For this review, take the finished solid that the model builds, in its own axes (mm). Face numbers are marked on the shaded views. A direction names the side the tool comes from. Coordinates: 2 decimals unless noted, no trailing zeros. Loops run counter-clockwise (first coordinate to the right, second up) from the corner with the lowest first, then second, coordinate; pieces in that order, holes last. Notation, with made-up numbers: (4, 47) -> (50, 47) arc R18 ccw to (50, 56) -> close; hole circle Ø4 at (9.5, -18.5). An arc over 180 degrees is marked (long way). Answer in a Markdown table with one row per item.
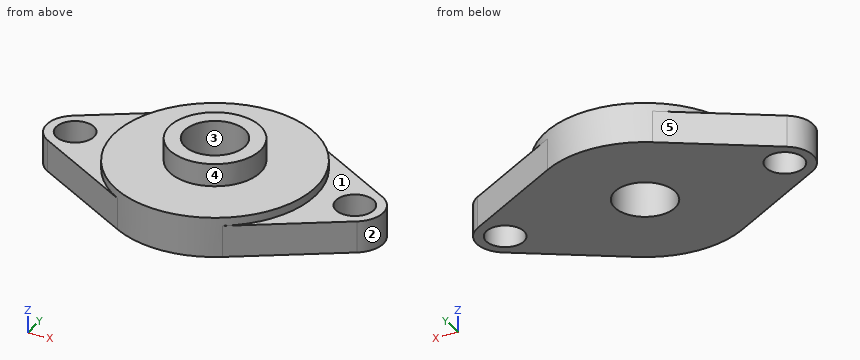
from build123d import *

# Parameters (mm, degrees)
SKETCH_1_R          = 3.75
SKETCH_1_R_2        = 2.5
SKETCH_1_R_3        = 13.3
SKETCH_1_R_4        = 4
EXTRUDE_1_DEPTH     = 4.2
SKETCH_1_3_R        = 13.3
SKETCH_1_3_R_2      = 4
EXTRUDE_2_DEPTH     = 8.3
CUT_EXTRUDE_START   = -3
SKETCH_2_R          = 13.3
SKETCH_2_R_2        = 6
CUT_EXTRUDE_1_DEPTH = 3


with BuildPart() as part:
    # Sketch 1 → Extrude 1 (new body)
    # profile 1 of 5: a face of its own
    with BuildSketch(Plane.XY):
        with Locations((-18.4, 0)):
            Circle(SKETCH_1_R)
        with Locations((-18.4, 0)):
            Circle(SKETCH_1_R_2, mode=Mode.SUBTRACT)
    # profile 2 of 5: a face of its own
    with BuildSketch(Plane.XY):
        with BuildLine():
            ThreePointArc((-6.90298913, -11.368321823), (-13.3, 0), (-6.90298913, 11.368321823))
            Line((-6.90298913, 11.368321823), (-20.346331522, 3.205353897))
            ThreePointArc((-20.346331522, 3.205353897), (-16.561011583, 3.26812203), (-14.65, 0))
            ThreePointArc((-14.65, 0), (-16.561011583, -3.26812203), (-20.346331522, -3.205353897))
            Line((-20.346331522, -3.205353897), (-6.90298913, -11.368321823))
        make_face()
    # profile 3 of 5: a face of its own
    with BuildSketch(Plane.XY):
        Circle(SKETCH_1_R_3)
        Circle(SKETCH_1_R_4, mode=Mode.SUBTRACT)
    # profile 4 of 5: a face of its own
    with BuildSketch(Plane.XY):
        with BuildLine():
            Line((20.346331522, 3.205353897), (6.90298913, 11.368321823))
            ThreePointArc((6.90298913, 11.368321823), (11.590939467, 6.522278918), (13.3, 0))
            ThreePointArc((13.3, 0), (11.590939467, -6.522278918), (6.90298913, -11.368321823))
            Line((6.90298913, -11.368321823), (20.346331522, -3.205353897))
            ThreePointArc((20.346331522, -3.205353897), (14.65, 0), (20.346331522, 3.205353897))
        make_face()
    # profile 5 of 5: a face of its own
    with BuildSketch(Plane.XY):
        with Locations((18.4, 0)):
            Circle(SKETCH_1_R)
        with Locations((18.4, 0)):
            Circle(SKETCH_1_R_2, mode=Mode.SUBTRACT)
    extrude(amount=EXTRUDE_1_DEPTH)

    # Sketch 1_3 → Extrude 2 (add)
    with BuildSketch(Plane.XY):
        with Locations(Location((0, 0, 0), (0, 0, 121.266654543))):
            Circle(SKETCH_1_3_R)
        Circle(SKETCH_1_3_R_2, mode=Mode.SUBTRACT)
    extrude(amount=EXTRUDE_2_DEPTH)

    # Sketch 2 → Cut-Extrude 1 (cut)
    with BuildSketch(Plane.XY.offset(8.3).offset(CUT_EXTRUDE_START)):
        with Locations(Location((0, 0, 0), (0, 0, 121.266654543))):
            Circle(SKETCH_2_R)
        Circle(SKETCH_2_R_2, mode=Mode.SUBTRACT)
    extrude(amount=CUT_EXTRUDE_1_DEPTH, mode=Mode.SUBTRACT)


solid = part.part
Item 1: Take a section at D-D, the plane x = -5.5. State the section outline as (y, z) points, and give its area (3 significant figures).
Worked answers:
| item | result |
|---|---|
| outline | (-12.11, 0) -> (12.11, 0) -> (12.11, 5.3) -> (2.4, 5.3) -> (2.4, 8.3) -> (-2.4, 8.3) -> (-2.4, 5.3) -> (-12.11, 5.3) -> close |
| area | 143 mm² |
Item 2: Take a section at B-B, the plane y = 0. State the section outline as (x, z) points, and give its area (3 significant figures).
Worked answers:
| item | result |
|---|---|
| outline | (-22.15, 0) -> (-20.9, 0) -> (-20.9, 4.2) -> (-22.15, 4.2) -> close; (-15.9, 0) -> (-4, 0) -> (-4, 8.3) -> (-6, 8.3) -> (-6, 5.3) -> (-13.3, 5.3) -> (-13.3, 4.2) -> (-15.9, 4.2) -> close; (4, 0) -> (15.9, 0) -> (15.9, 4.2) -> (13.3, 4.2) -> (13.3, 5.3) -> (6, 5.3) -> (6, 8.3) -> (4, 8.3) -> close; (20.9, 0) -> (22.15, 0) -> (22.15, 4.2) -> (20.9, 4.2) -> close |
| area | 143 mm² |
Item 3: Take a section at A-A, the plane x = 0. State the section outline as (y, z) points.
Worked answers:
| item | result |
|---|---|
| outline | (-13.3, 0) -> (-4, 0) -> (-4, 8.3) -> (-6, 8.3) -> (-6, 5.3) -> (-13.3, 5.3) -> close; (4, 0) -> (13.3, 0) -> (13.3, 5.3) -> (6, 5.3) -> (6, 8.3) -> (4, 8.3) -> close |
Item 4: For the marked faces 4 and 5, list the 3-axis set-ups (+Z, -Z, +X, -X, +Y, -Y) from which the entire face can be reached by the end or side of a thin tool; tool diameter is ignored.
Worked answers:
| item | result |
|---|---|
| face 4 | +Z |
| face 5 | +Z, -Z, -X, +Y |
Item 5: Insertion check: pin 1 (4 mm diameter, centred on y = -1.5, z = 5, fed in from -X); pin 2 (8 mm diameter, centred on x = -18.4, y = 0, fed in from +Z); pin 3 (3 mm diameter, centred on y = -8.5, z = 3.5, fed in from -X); pin 4 (4.5 mm diameter, centred on x = 18.4, y = 0, fed in from -Z). Each pin has a flat end and moves straight along its axis. Give the tip position at first contact, or say it passes through.
Worked answers:
| item | result |
|---|---|
| pin 1 | x = -22.15 |
| pin 2 | z = 4.2 |
| pin 3 | x = -14.1 |
| pin 4 | through |
Item 6: For L1, parallel to Y at x = 0, z = 6.75; L2, parallel to X at y = -1.25, z = 3.5; L3, parallel to X at y = 0.25, z = 5.25, list the stretches that pass through material, from the lowest coordinate up.
Worked answers:
| item | result |
|---|---|
| L1 | -6 to -4, 4 to 6 |
| L2 | -21.94 to -20.57, -16.23 to -3.8, 3.8 to 16.23, 20.57 to 21.94 |
| L3 | -13.3 to -3.99, 3.99 to 13.3 |
Item 7: The part is to be moulded in two halves that separate along Y. For the marked faces 1, 2 and 3, say which applies: +Y half, -Y half, draft (parallel to the pull), parting line (faces both ways), or undercut.
Worked answers:
| item | result |
|---|---|
| face 1 | draft |
| face 2 | parting line |
| face 3 | undercut |
Item 8: Take a section at C-C, the plane z = 2.75. State the section outline as (x, y) points, and give its area (3 significant figures).
Worked answers:
| item | result |
|---|---|
| outline | (-20.35, -3.21) -> (-6.9, -11.37) arc R13.3 ccw to (6.9, -11.37) -> (20.35, -3.21) arc R3.75 ccw to (20.35, 3.21) -> (6.9, 11.37) arc R13.3 ccw to (-6.9, 11.37) -> (-20.35, 3.21) arc R3.75 ccw to start; hole circle Ø5 at (-18.4, 0); hole circle Ø8 at (0, 0); hole circle Ø5 at (18.4, 0) |
| area | 669 mm² |
